For this review, take the finished solid that the model builds, in its own axes (mm). A direction names the side the tool comes from. Round coordinates to 2 decimals unless told otherwise and drop trailing zeros. Write each loop counter-clockwise with the first axis right and the second up, starting at its lowest first coordinate (ties: lowest second). Pieces come first, ordered by that corner, then holes. Notation, with made-up numbers: M 19.5,-11.75 L 28.5,-11.75 A26 ccw 28.5,16.25 Z; hole C -20.5,-0.75 d11. An arc over 180 degrees is marked long. Use one line per item in the form item = value. Start each with the question number.
Item 1: For P1, Ø15, axis at x = 10, z = 35, coming from the +Y side; P2, Ø1.2, axis at x = -0.5, y = 29, coming from the +Z side; P3, Ø6.5, axis at x = -23.55, y = -23.55, coming from the +Z side; P4, Ø4, axis at x = 23.55, y = 23.55, coming from the -Z side, all flat-tipped, find the tip position at first contact; note any pin that passes through.
Item 2: For line 1 (Y direction, x = 23.55, z = 73.95); line 2 (Z direction, x = 21, y = 0.5); line 3 (Y direction, x = -2, z = 54.5), list the stretches that pass through material, from the lowest coordinate up. Write a range as [from, to].
Item 3: Draft analysis for pull direction X (two halves, no side actions). For faces 6 (the cylindrical face through (1.5, 2.8, 0.2)), 7 (the cylindrical face through (-16.7, 26.77, 36)), 8 (the flat face through (6, 0, 0)), state which applies: released by +X, released by -X, zero draft, split by the parting line, or undercut.
Item 4: Add section C-C (x = 11). State the section outline as (y, z) points, and give its area (3 significant figures).
Item 5: Add section A-A (y = 0). State the section outline as (x, z) points (3 decimals).
Item 6: Add section D-D (x = -15.5). State the section outline as (y, z) points, and give its area (3 significant figures).
Item 7: For faces 1 (the flat face through (21, 22, 71)), 2 (the cylindrical face through (-19.7, 19.63, 36)), 3 (the flat face through (-0.4, 19.2, 76)), 4 (the flat face through (21, -22, 71)), 5 (the cylindrical face through (-16.7, -26.77, 36)), list the 3-axis set-ups (+Z, -Z, +X, -X, +Y, -Y) from which the entire face can be reached by the end or side of a thin tool; tool diameter is ignored.
from build123d import *

# Parameters (mm, degrees)
SKETCH_1_W                  = 56.4
SKETCH_1_H                  = 56.4
EXTRUDE_1_DEPTH             = 76
SKETCH_2_R                  = 19.05
EXTRUDE_2_DEPTH             = 1.6
SKETCH_3_R                  = 3.175
EXTRUDE_3_DEPTH             = 19
SKETCH_4_R                  = 3.175
CUT_EXTRUDE_1_DEPTH         = 0.5
SKETCH_6_W                  = 10
SKETCH_6_H                  = 10
CUT_EXTRUDE_2_DEPTH         = 71
PATTERN_LINEAR_1_COUNT      = 2
PATTERN_LINEAR_1_PITCH      = 46.4
PATTERN_LINEAR_1_COUNT_DIR2 = 2
PATTERN_LINEAR_1_PITCH_DIR2 = 46.4
FILLET_1_R                  = 5
SKETCH_7_R                  = 2.5
CUT_EXTRUDE_3_DEPTH         = 71
PATTERN_LINEAR_2_COUNT      = 2
PATTERN_LINEAR_2_PITCH      = 47.1
PATTERN_LINEAR_2_COUNT_DIR2 = 2
PATTERN_LINEAR_2_PITCH_DIR2 = 47.1
FILLET_2_R                  = 3
FILLET_3_R                  = 0.5
SKETCH_8_W                  = 10
SKETCH_8_H                  = 10
EXTRUDE_4_DEPTH             = 2
FILLET_4_R                  = 0.5


with BuildPart() as part:
    # Эскиз1 → Бобышка-Вытянуть1 (new body)
    with BuildSketch(Plane.XY):
        Rectangle(SKETCH_1_W, SKETCH_1_H)
    extrude(amount=EXTRUDE_1_DEPTH)

    # Эскиз2 → Бобышка-Вытянуть2 (add)
    with BuildSketch(Plane.XY.offset(76)):
        Circle(SKETCH_2_R)
    extrude(amount=EXTRUDE_2_DEPTH)

    # Эскиз3 → Бобышка-Вытянуть3 (add)
    with BuildSketch(Plane.XY.offset(77.6)):
        Circle(SKETCH_3_R)
    extrude(amount=EXTRUDE_3_DEPTH)

    # Эскиз4 → Вырез-Вытянуть1 (cut)
    with BuildSketch(Plane(origin=(0, 0, 0), x_dir=(-1, 0, 0), z_dir=(0, 0, -1))):
        with Locations(Location((0, 0, 0), (0, 0, 180))):
            Circle(SKETCH_4_R)
    extrude(amount=-CUT_EXTRUDE_1_DEPTH, mode=Mode.SUBTRACT)

    # Эскиз6 → Вырез-Вытянуть2 (cut)
    with BuildSketch(Plane(origin=(0, 0, 0), x_dir=(-1, 0, 0), z_dir=(0, 0, -1))):
        with Locations((-23.2, 23.2)):
            Rectangle(SKETCH_6_W, SKETCH_6_H)
    cut_extrude_2 = extrude(amount=-CUT_EXTRUDE_2_DEPTH, mode=Mode.SUBTRACT)

    # Линейный массив1: Cut-Extrude 2 2 × 2
    with Locations(*[(-i * PATTERN_LINEAR_1_PITCH, -j * PATTERN_LINEAR_1_PITCH_DIR2, 0) for i in range(PATTERN_LINEAR_1_COUNT) for j in range(PATTERN_LINEAR_1_COUNT_DIR2) if (i, j) != (0, 0)]):
        add(cut_extrude_2, mode=Mode.SUBTRACT)

    # Скругление1
    fillet_1_edges = [part.edges().sort_by_distance(p)[0] for p in [
        (-28.2, 18.2, 35.5),
        (-28.2, -18.2, 35.5),
        (-18.2, -28.2, 35.5),
        (18.2, -28.2, 35.5),
        (28.2, -18.2, 35.5),
        (28.2, 18.2, 35.5),
        (-18.2, 28.2, 35.5),
        (18.2, 28.2, 35.5),
        (18.2, -18.2, 35.5),
        (-18.2, -18.2, 35.5),
        (-18.2, 18.2, 35.5),
        (18.2, 18.2, 35.5),
    ]]
    fillet(fillet_1_edges, radius=FILLET_1_R - 0.0001)  # a hair under: the kernel refuses the full size

    # Эскиз7 → Вырез-Вытянуть3 (cut)
    with BuildSketch(Plane.XY.offset(76)):
        with Locations((-23.55, 23.55)):
            Circle(SKETCH_7_R)
    cut_extrude_3 = extrude(amount=-CUT_EXTRUDE_3_DEPTH, mode=Mode.SUBTRACT)

    # Линейный массив2: Cut-Extrude 3 2 × 2
    with Locations(*[(i * PATTERN_LINEAR_2_PITCH, -j * PATTERN_LINEAR_2_PITCH_DIR2, 0) for i in range(PATTERN_LINEAR_2_COUNT) for j in range(PATTERN_LINEAR_2_COUNT_DIR2) if (i, j) != (0, 0)]):
        add(cut_extrude_3, mode=Mode.SUBTRACT)

    # Скругление2
    fillet_2_edges = [part.edges().sort_by_distance(p)[0] for p in [
        (28.2, -28.2, 73.5),
        (-28.2, -28.2, 73.5),
        (-28.2, 28.2, 73.5),
        (28.2, 28.2, 73.5),
    ]]
    fillet(fillet_2_edges, radius=FILLET_2_R)

    # Скругление3
    fillet_3_edges = [part.edges().sort_by_distance(p)[0] for p in [
        (-3.175, 0, 96.6),
    ]]
    fillet(fillet_3_edges, radius=FILLET_3_R)

    # Эскиз8 → Бобышка-Вытянуть4 (add)
    with BuildSketch(Plane(origin=(0, 28.2, 0), x_dir=(1, 0, 0), z_dir=(0, 1, 0))):
        with Locations((0, -6)):
            Rectangle(SKETCH_8_W, SKETCH_8_H)
    extrude(amount=EXTRUDE_4_DEPTH)

    # Скругление4
    fillet_4_edges = [part.edges().sort_by_distance(p)[0] for p in [
        (5, 30.2, 6),
        (0, 30.2, 1),
        (-5, 30.2, 6),
        (0, 30.2, 11),
    ]]
    fillet(fillet_4_edges, radius=FILLET_4_R)


solid = part.part
Calculated:
q1.P1 = 28.2
q1.P2 = 11
q1.P3 = 76
q1.P4 = through
q2.line_1 = [-28.2, -26.05], [-21.05, 21.05], [26.05, 28.2]
q2.line_2 = [0, 76]
q2.line_3 = [-28.2, 28.2]
q3.face_6 = undercut
q3.face_7 = released by -X
q3.face_8 = zero draft
q4.outline = M -28.2,0 L 28.2,0 L 28.2,76 L 15.55,76 L 15.55,77.6 L -15.55,77.6 L -15.55,76 L -28.2,76 Z
q4.area = 4,340 mm^2
q5.outline = M -28.2,0 L -3.175,0 L -3.175,0.5 L 3.175,0.5 L 3.175,0 L 28.2,0 L 28.2,76 L 19.05,76 L 19.05,77.6 L 3.175,77.6 L 3.175,96.1 A0.5 ccw 2.675,96.6 L -2.675,96.6 A0.5 ccw -3.175,96.1 L -3.175,77.6 L -19.05,77.6 L -19.05,76 L -28.2,76 Z
q6.outline = M -28.2,71 L -27.64,71 L -27.64,0 L 27.64,0 L 27.64,71 L 28.2,71 L 28.2,76 L 11.07,76 L 11.07,77.6 L -11.07,77.6 L -11.07,76 L -28.2,76 Z
q6.area = 4,240 mm^2
q7.face_1 = -Z, +X, +Y
q7.face_2 = -Z, -X, +Y
q7.face_3 = +Z
q7.face_4 = -Z, +X, -Y
q7.face_5 = -Z, -X, -Y
